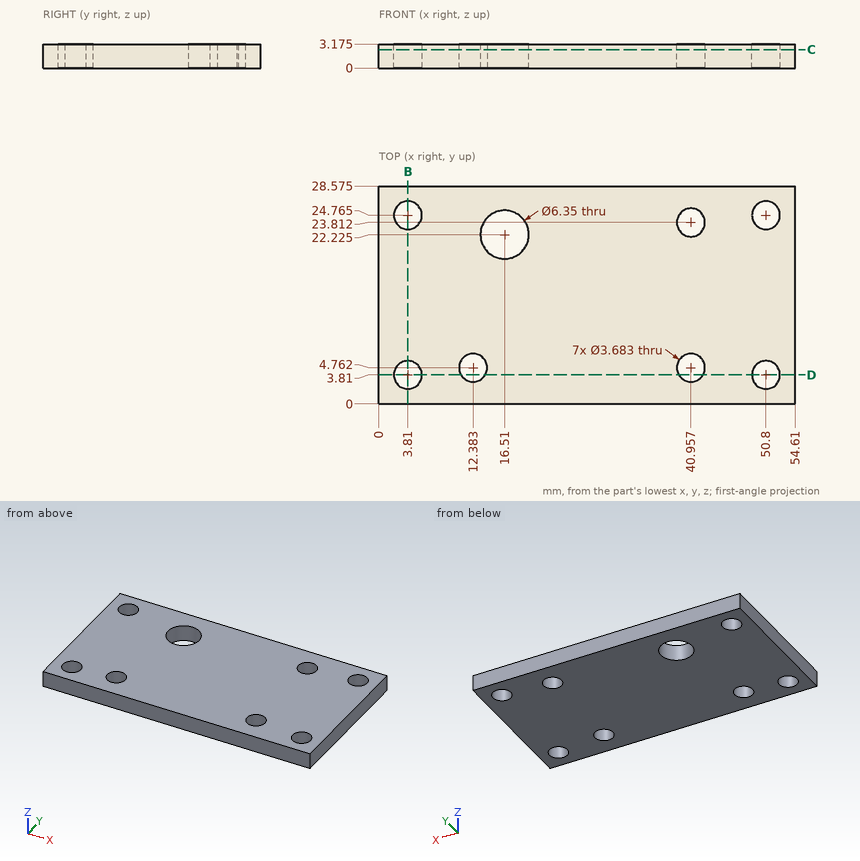
Part print with two shaded views. Sizes in mm from the minimum x, y, z corner. Round coordinates to 2 decimals unless told otherwise and drop trailing zeros. Order: outer loops, then holes, each group sorted by start corner. A loop starts at its lowest first (then second) coordinate and runs counter-clockwise, first axis right, second up. Notation, with made-up numbers: (19, 81.25) -> (68, 81.25) arc R16 cw to (68, 104.25) -> close; hole circle Ø5 at (-25.75, 31). An arc over 180 degrees is marked (long way). Use one line per item in the form item = value.
Item 1: Cut at C-C, the plane z = 2.45. Give the number of separate pieces and of enclosed holes in the cut face, and give its area (3 significant figures).
Returned:
separate_pieces = 1
enclosed_holes = 8
area = 1,450 mm^2
Item 2: Cut at D-D, the plane y = 3.81. Write the cut outline in (x, z) (1 decimal).
Returned:
outline = (0, 0) -> (2, 0) -> (2, 3.2) -> (0, 3.2) -> close; (5.7, 0) -> (10.8, 0) -> (10.8, 3.2) -> (5.7, 3.2) -> close; (14, 0) -> (39.4, 0) -> (39.4, 3.2) -> (14, 3.2) -> close; (42.5, 0) -> (49, 0) -> (49, 3.2) -> (42.5, 3.2) -> close; (52.6, 0) -> (54.6, 0) -> (54.6, 3.2) -> (52.6, 3.2) -> close
Item 3: Cut at B-B, the plane x = 3.81. Write the cut outline in (y, z) (1 decimal).
Returned:
outline = (0, 0) -> (2, 0) -> (2, 3.2) -> (0, 3.2) -> close; (5.7, 0) -> (22.9, 0) -> (22.9, 3.2) -> (5.7, 3.2) -> close; (26.6, 0) -> (28.6, 0) -> (28.6, 3.2) -> (26.6, 3.2) -> close
Item 4: Drill centre lines: line 1 (Y direction, x = 50.8, z = 1.2) (1 decimal); line 2 (Y direction, x = 5.5, z = 1.5) (1 decimal); line 3 (X direction, y = 19.5, z = 0.6). Where is each one in solid material? Low to high.
Returned:
line_1 = 0 to 2, 5.7 to 22.9, 26.6 to 28.6
line_2 = 0 to 3.1, 4.5 to 24, 25.5 to 28.6
line_3 = 0 to 14.88, 18.14 to 54.61
